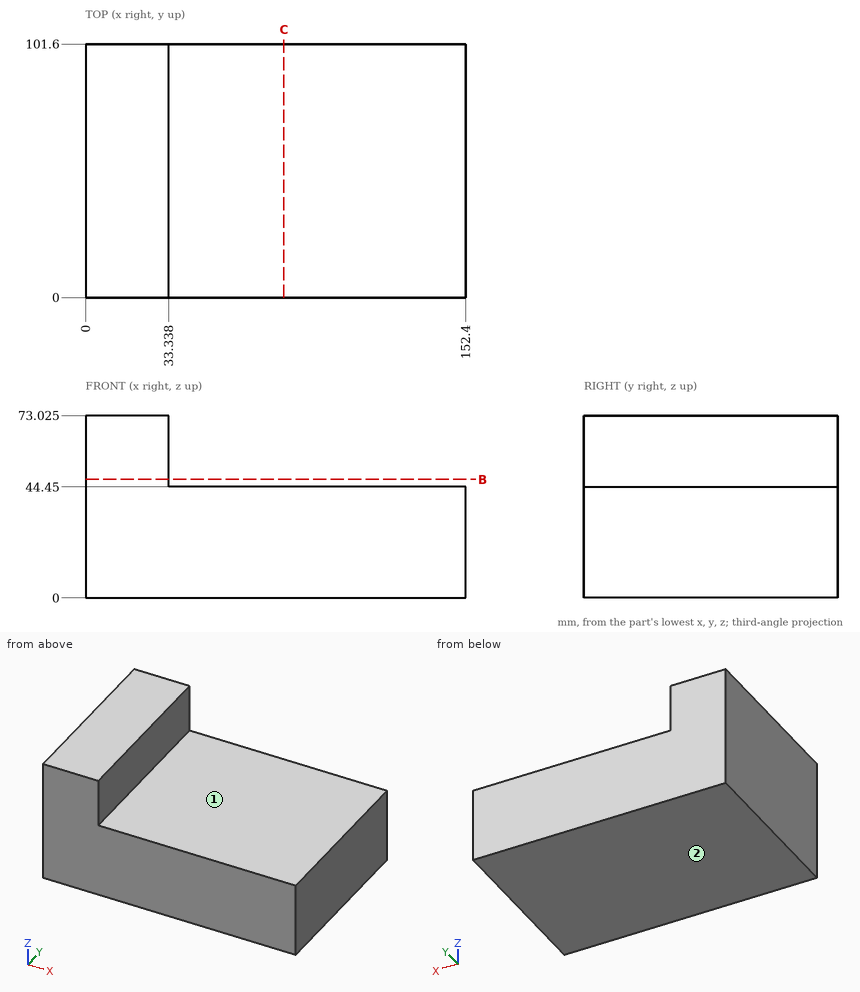
Here's the drawing with two shaded views (mm, measured from the low corner). I have some questions. A direction names the side the tool comes from. Coordinates: 2 decimals unless noted, no trailing zeros. Loops run counter-clockwise (first coordinate to the right, second up) from the corner with the lowest first, then second, coordinate; pieces in that order, holes last.
Item 1: Please list where these lines run through material, in increasing order: L1, parallel to X at y = 22, z = 53; L2, parallel to Z at x = 44, y = 8.
Answers below:
L1: x = 0 to 33.34
L2: z = 0 to 44.45
Item 2: Which directions (+Z, -Z, +X, -X, +Y, -Y) give clear straight access to the entire face, cutting with the end or side of a thin tool? Please do the marked faces 1 and 2.
Answers below:
face 1: +Z, +X, +Y, -Y
face 2: -Z, +X, -X, +Y, -Y
Item 3: Suppose I cut it at B-B (z = 47.5). Please give me the cut outline in (x, y), then the cut area to 3 significant figures.
Answers below:
outline: (0, 0) - (33.34, 0) - (33.34, 101.6) - (0, 101.6) - close
area: 3,390 mm2
Item 4: Suppose I cut it at C-C (x = 79.5). Please give me the cut outline in (y, z), then the cut area to 3 significant figures.
Answers below:
outline: (0, 0) - (101.6, 0) - (101.6, 44.45) - (0, 44.45) - close
area: 4,520 mm2
Item 5: I'm going to push flat-ended pins straight in: pin 1 (6 mm diameter, centred on x = 33.5, y = 25, fed in from +Z) (1 decimal); pin 2 (14.5 mm diameter, centred on y = 65.5, z = 60, fed in from +X). Where does each tip first touch, or does it pass through?
Answers below:
pin 1: stops at z = 73
pin 2: stops at x = 33.34
